```python
from build123d import *

# Parameters (mm, degrees)
EXTRUDE_1_DEPTH     = 8
SKETCH_2_R          = 2.5
CUT_EXTRUDE_1_DEPTH = 6
SKETCH_3_R          = 2.5
CUT_EXTRUDE_2_DEPTH = 6
FILLET_1_R          = 10
SKETCH_4_W          = 39
SKETCH_4_H          = 48
SKETCH_4_W_2        = 5
SKETCH_4_H_2        = 5
CUT_EXTRUDE_3_DEPTH = 21
SKETCH_5_R          = 5
EXTRUDE_2_DEPTH     = 8
FILLET_2_R          = 4
FILLET_3_R          = 4
SKETCH_6_R          = 2.5
CUT_EXTRUDE_4_DEPTH = 6
SKETCH_7_R          = 2.5
CUT_EXTRUDE_5_DEPTH = 6


with BuildPart() as part:
    # Эскиз1 → Бобышка-Вытянуть1 (new body)
    with BuildSketch(Plane.XY):
        Polygon((-23.5, 62.203361065), (-23.5, 77.203361065), (-31.5, 77.203361065), (-31.5, -77.203361065), (31.5, -77.203361065), (31.5, 77.203361065), (23.5, 77.203361065), (23.5, 62.203361065), align=None)
    extrude(amount=EXTRUDE_1_DEPTH)

    # Эскиз2 → Вырез-Вытянуть1 (cut)
    with BuildSketch(Plane(origin=(0, 77.203361065, 0), x_dir=(1, 0, 0), z_dir=(0, 1, 0))):
        with Locations(Location((-27.5, -4, 0), (0, 0, 180))):
            Circle(SKETCH_2_R)
        with Locations((27.5, -4)):
            Circle(SKETCH_2_R)
    extrude(amount=-CUT_EXTRUDE_1_DEPTH, mode=Mode.SUBTRACT)

    # Эскиз3 → Вырез-Вытянуть2 (cut)
    with BuildSketch(Plane.XY.offset(8)):
        with Locations((-24.5, 55.203361065)):
            Circle(SKETCH_3_R)
        with Locations((24.5, 55.203361065)):
            Circle(SKETCH_3_R)
        with Locations((24.5, -2.796638935)):
            Circle(SKETCH_3_R)
        with Locations((-24.5, -2.796638935)):
            Circle(SKETCH_3_R)
    extrude(amount=-CUT_EXTRUDE_2_DEPTH, mode=Mode.SUBTRACT)

    # Скругление1
    fillet_1_edges = [part.edges().sort_by_distance(p)[0] for p in [
        (-23.5, 62.203361065, 4),
        (23.5, 62.203361065, 4),
    ]]
    fillet(fillet_1_edges, radius=FILLET_1_R)

    # Эскиз4 → Вырез-Вытянуть3 (cut)
    with BuildSketch(Plane.XY.offset(8)):
        with Locations((0, 26.203361065)):
            Rectangle(SKETCH_4_W, SKETCH_4_H)
        with Locations((-22, 26.203361065)):
            Rectangle(SKETCH_4_W_2, SKETCH_4_H)
        with Locations((0, 52.703361065)):
            Rectangle(SKETCH_4_W, SKETCH_4_H_2)
        with Locations((22, 26.203361065)):
            Rectangle(SKETCH_4_W_2, SKETCH_4_H)
        with Locations((0, -0.296638935)):
            Rectangle(SKETCH_4_W, SKETCH_4_H_2)
    extrude(amount=-CUT_EXTRUDE_3_DEPTH, mode=Mode.SUBTRACT)

    # Эскиз5 → Бобышка-Вытянуть2 (add)
    with BuildSketch(Plane(origin=(0, 0, 0), x_dir=(-1, 0, 0), z_dir=(0, 0, -1))):
        with Locations((-27.95, 47.203361065)):
            Circle(SKETCH_5_R)
        with Locations((-27.95, 28.403361065)):
            Circle(SKETCH_5_R)
        with Locations((27.95, 28.403361065)):
            Circle(SKETCH_5_R)
        with Locations((27.95, 47.203361065)):
            Circle(SKETCH_5_R)
    extrude(amount=-EXTRUDE_2_DEPTH)

    # Скругление2
    fillet_2_edges = [part.edges().sort_by_distance(p)[0] for p in [
        (-19.5, 2.203361065, 4),
        (-19.5, 50.203361065, 4),
        (19.5, 50.203361065, 4),
        (19.5, 2.203361065, 4),
    ]]
    fillet(fillet_2_edges, radius=FILLET_2_R)

    # Скругление3
    fillet_3_edges = [part.edges().sort_by_distance(p)[0] for p in [
        (-24.5, 32.0224079, 4),
        (-24.5, 24.784314229, 4),
        (-24.5, 43.584314229, 4),
        (-23.95, 50.203361065, 4),
        (-19.5, 55.203361065, 4),
        (24.5, 32.0224079, 4),
        (24.5, 24.784314229, 4),
        (24.5, 43.584314229, 4),
        (19.5, 55.203361065, 4),
        (23.95, 50.203361065, 4),
        (24.5, 2.203361065, 4),
        (19.5, -2.796638935, 4),
        (-19.5, -2.796638935, 4),
        (-24.5, 2.203361065, 4),
    ]]
    fillet(fillet_3_edges, radius=FILLET_3_R)

    # Эскиз6 → Вырез-Вытянуть4 (cut)
    with BuildSketch(Plane(origin=(0, 0, 0), x_dir=(-1, 0, 0), z_dir=(0, 0, -1))):
        with Locations((-27.95, 47.203361065)):
            Circle(SKETCH_6_R)
        with Locations((27.95, 47.203361065)):
            Circle(SKETCH_6_R)
        with Locations((27.95, 28.403361065)):
            Circle(SKETCH_6_R)
        with Locations((-27.95, 28.403361065)):
            Circle(SKETCH_6_R)
    extrude(amount=-CUT_EXTRUDE_4_DEPTH, mode=Mode.SUBTRACT)

    # Эскиз7 → Вырез-Вытянуть5 (cut)
    with BuildSketch(Plane.ZY.offset(31.5)):
        with Locations((4, 62.203361065)):
            Circle(SKETCH_7_R)
    cut_extrude_5 = extrude(amount=-CUT_EXTRUDE_5_DEPTH, mode=Mode.SUBTRACT)

    # Зеркальное отражение1: Вырез-Вытянуть5 across plane
    add(cut_extrude_5.mirror(Plane(origin=(0, 0, 0), x_dir=(0, 0, 1), z_dir=(1, 0, 0))), mode=Mode.SUBTRACT)


solid = part.part
```
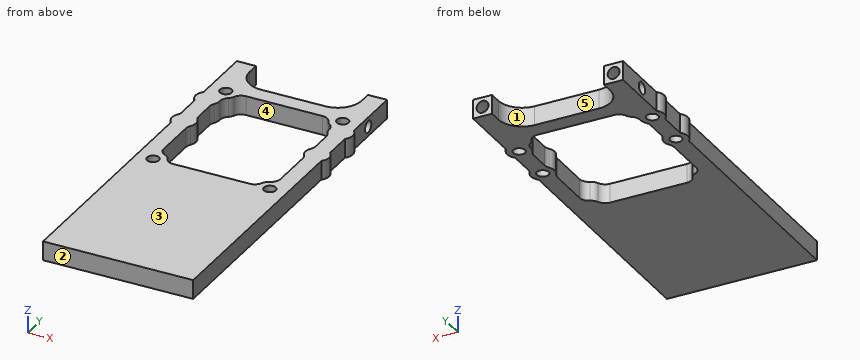
Can you work these out from the model? Positions are in its coordinate system, mm. Face numbers are marked on the shaded views. A direction names the side the tool comes from. Give positions to 0.01 mm unless a question says otherwise; leave off trailing zeros. Loops run counter-clockwise (first coordinate to the right, second up) from the corner with the lowest first, then second, coordinate; pieces in that order, holes last. Notation, with made-up numbers: M 72,-10 L 88,-10 A21 ccw 88,20 Z; hole C 26,13 d1. An arc over 180 degrees is marked long. Answer in a Markdown table with one row per item.
1. Thinking about a two-plate mould opening in X: for the marked faces 1 and 2, which applies, released by +X, released by -X, zero draft, split by the parting line, or undercut?
Taken from the geometry:
| item | result |
|---|---|
| face 1 | undercut |
| face 2 | zero draft |
2. For pin 1 Ø4.5 at (y, z) = (62.2, 4) entering from +X; pin 2 Ø4 at (y, z) = (36.5, 4.5) entering from -X; pin 3 Ø2.5 at (y, z) = (-29, 3.5) entering from +X, each with a flat end and sliding along its axis, tell me the tip position at first contact or that it passes through.
Taken from the geometry:
| item | result |
|---|---|
| pin 1 | stops at x = 25.5 |
| pin 2 | stops at x = -31.5 |
| pin 3 | stops at x = 31.5 |
3. Suppose I cut it at A-A on x = 10. Write out the boundary of the cut face in (y, z), plus the area to 3 significant figures.
Taken from the geometry:
| item | result |
|---|---|
| outline | M -77.2,0 L -2.8,0 L -2.8,8 L -77.2,8 Z; M 55.2,0 L 62.2,0 L 62.2,8 L 55.2,8 Z |
| area | 651 mm² |
4. Suppose I cut it at C-C on z = 4. Count the separate pieces of the cut face and the enclosed holes in it, plus the area to 3 significant figures.
Taken from the geometry:
| item | result |
|---|---|
| separate pieces | 1 |
| enclosed holes | 9 |
| area | 6,110 mm² |
5. If I drill on line 1 along Y through (x, z) = (-4.5, 4.75); line 2 along Y through (x, z) = (-26, 3.75); line 3 along Z through (x, y) = (27.5, 73), over which ranges is the centre line in solid material (lowest first)?
Taken from the geometry:
| item | result |
|---|---|
| line 1 | y = -77.2 to -2.8, 55.2 to 62.2 |
| line 2 | y = -77.2 to -4.8, -0.8 to 26.84, 29.97 to 45.64, 48.77 to 53.2, 57.2 to 59.72, 64.69 to 71.2 |
| line 3 | z = 0 to 1.5, 6.5 to 8 |
6. Which directions (+Z, -Z, +X, -X, +Y, -Y) give clear straight access to the entire face, cutting with the end or side of a thin tool? Please do the marked faces 3, 4 and 5.
Taken from the geometry:
| item | result |
|---|---|
| face 3 | +Z, +X, -X, +Y, -Y |
| face 4 | +Z, -Z |
| face 5 | +Z, -Z, +Y |
7. Suppose I cut it at B-B on y = -28.5. Write out the boundary of the cut face in (x, z).
Taken from the geometry:
| item | result |
|---|---|
| outline | M -31.5,0 L 31.5,0 L 31.5,8 L -31.5,8 Z |
